Geometry: final body of the model. Coordinates: model frame, mm. A direction names the side the tool comes from. Coordinates: 2 decimals unless noted, no trailing zeros. Write each loop counter-clockwise with the first axis right and the second up, starting at its lowest first coordinate (ties: lowest second). Pieces come first, ordered by that corner, then holes. Notation, with made-up numbers: (-16.5, -40) - (3.5, -40) arc R12 cw to (3.5, -29) - close; hole circle Ø3 at (60.25, 70). An arc over 180 degrees is marked (long way). Answer as a JSON object with one key per item and string values. Group by question number.
Item 1: Mould query, pull axis Z, two halves, no side actions, for faces 1 (the cylindrical face through (68.86, -22.46, -11.22)), 2 (the flat face through (33, 1, 0)), 3 (the cylindrical face through (-7.464, -22.465, -13.214)), 4 (the flat face through (5, -12, -10)). Classes: pulls with the +Z half, pulls with the -Z half, needs draft (parallel to the pull), parting line crosses it, or undercut.
Item 2: Section D-D on z = -17.25. Return loops of the section in (x, y).
Item 3: Set-up query: faces 5 (the flat face through (-0.5, -20, -10.1)), 6 (the flat face through (-0.7, -25, -10.1)), 7 (the flat face through (60.5, -20, -9.9)), 8 (the flat face through (30, 0, -10)). Return all of +Z, -Z, +X, -X, +Y, -Y with unobstructed straight access to the full face (end or side cutting, diameter ignored); none if empty.
Item 4: First-contact query: pin 1 Ø6.5 at (x, z) = (65, -10) entering from -Y; pin 2 Ø3 at (y, z) = (-7.5, -13.5) entering from +X; pin 3 Ø10 at (x, z) = (21, -6.5) entering from -Y; pin 4 Ø3 at (y, z) = (-17.5, -5) entering from -X. Flat tips, straight axial feed; report the tip coordinate or a pass-through.
Item 5: Line query: line 1 along X through (y, z) = (-23.5, -10); line 2 along X through (y, z) = (-23, -3.5); line 3 along X through (y, z) = (-11, -5.5). Output: solid intervals per line, ascending. Write a range as from..to.
Item 6: Section B-B on z = -10. Return loops of the section in (x, y), and give its area (3 significant figures).
Item 7: Section A-A on x = -5. Return loops of the section in (y, z).
Item 8: Section C-C on y = -6. Return loops of the section in (x, z).
```python
from build123d import *

# Parameters (mm, degrees)
SKETCH1_W           = 60
SKETCH1_H           = 20
BOSS_EXTRUDE1_DEPTH = 5
SKETCH2_W           = 5
SKETCH2_H           = 20
BOSS_EXTRUDE2_DEPTH = 25
SKETCH3_W           = 20
SKETCH3_H           = 5
BOSS_EXTRUDE3_DEPTH = 10
SKETCH4_W           = 20
SKETCH4_H           = 5
BOSS_EXTRUDE4_DEPTH = 10
SKETCH5_R           = 4.05
CUT_EXTRUDE1_DEPTH  = 20


with BuildPart() as part:
    # Sketch1 → Boss-Extrude1 (new body)
    with BuildSketch(Plane(origin=(0, 0, 0), x_dir=(1, 0, 0), z_dir=(0, 1, 0))):
        with Locations((30, 10)):
            Rectangle(SKETCH1_W, SKETCH1_H)
    extrude(amount=BOSS_EXTRUDE1_DEPTH)

    # Sketch2 → Boss-Extrude2 (add)
    with BuildSketch(Plane.XZ):
        with Locations((2.5, -10)):
            Rectangle(SKETCH2_W, SKETCH2_H)
        with Locations((57.5, -10)):
            Rectangle(SKETCH2_W, SKETCH2_H)
    extrude(amount=BOSS_EXTRUDE2_DEPTH)

    # Sketch3 → Boss-Extrude3 (add)
    with BuildSketch(Plane(origin=(60, 0, 0), x_dir=(0, 0, -1), z_dir=(1, 0, 0))):
        with Locations((10, -22.5)):
            Rectangle(SKETCH3_W, SKETCH3_H)
    extrude(amount=BOSS_EXTRUDE3_DEPTH)

    # Sketch4 → Boss-Extrude4 (add)
    with BuildSketch(Plane.ZY):
        with Locations((-10, -22.5)):
            Rectangle(SKETCH4_W, SKETCH4_H)
    extrude(amount=BOSS_EXTRUDE4_DEPTH)

    # Sketch5 → Cut-Extrude1 (cut)
    with BuildSketch(Plane(origin=(0, -20, 0), x_dir=(1, 0, 0), z_dir=(0, 1, 0))):
        with BuildLine():
            ThreePointArc((60.95, 10), (65, 5.95), (69.05, 10))
            Line((69.05, 10), (60.95, 10))
        make_face()
        with BuildLine():
            Line((60.95, 10), (69.05, 10))
            ThreePointArc((69.05, 10), (65, 14.05), (60.95, 10))
        make_face()
        with Locations(Location((-5, 10, 0), (0, 0, 270))):
            Circle(SKETCH5_R)
    extrude(amount=-CUT_EXTRUDE1_DEPTH, mode=Mode.SUBTRACT)


solid = part.part
```
Checks:
{
 "1": {"face 1": "undercut", "face 2": "pulls with the +Z half", "face 3": "undercut", "face 4": "needs draft"},
 "2": {"outline": "(-10, -25) - (5, -25) - (5, 0) - (55, 0) - (55, -25) - (70, -25) - (70, -20) - (60, -20) - (60, 5) - (0, 5) - (0, -20) - (-10, -20) - close"},
 "3": {"face 5": "+Z, -Z, -X, +Y", "face 6": "+Z, -Z, +X, -X, -Y", "face 7": "+Z, -Z, +X, +Y", "face 8": "+Z, -Z, -Y"},
 "4": {"pin 1": "through", "pin 2": "x = 60", "pin 3": "y = 0", "pin 4": "x = 0"},
 "5": {"line 1": "-10..-9.05, -0.95..5, 55..60.95, 69.05..70", "line 2": "-10..5, 55..70", "line 3": "0..5, 55..60"},
 "6": {"outline": "(-10, -25) - (-9.05, -25) - (-9.05, -20) - (-10, -20) - close; (-0.95, -25) - (5, -25) - (5, 0) - (55, 0) - (55, -25) - (60.95, -25) - (60.95, -20) - (60, -20) - (60, 5) - (0, 5) - (0, -20) - (-0.95, -20) - close; (69.05, -25) - (70, -25) - (70, -20) - (69.05, -20) - close", "area": "569 mm^2"},
 "7": {"outline": "(-25, -20) - (-20, -20) - (-20, -14.05) - (-25, -14.05) - close; (-25, -5.95) - (-20, -5.95) - (-20, 0) - (-25, 0) - close"},
 "8": {"outline": "(0, -20) - (5, -20) - (5, 0) - (0, 0) - close; (55, -20) - (60, -20) - (60, 0) - (55, 0) - close"}
}
